CAD build for the part. Positions are in the model's coordinates, mm. Face numbers are marked on the shaded views. A direction names the side the tool comes from. Coordinates: 2 decimals unless noted, no trailing zeros. Loops run counter-clockwise (first coordinate to the right, second up) from the corner with the lowest first, then second, coordinate; pieces in that order, holes last. Notation, with made-up numbers: (-17.75, 53.5) -> (41.25, 53.5) arc R21 cw to (41.25, 92.5) -> close; hole circle Ø1 at (68.5, 66). An arc over 180 degrees is marked (long way). Write each question's results on one line, items separated by ' | '.
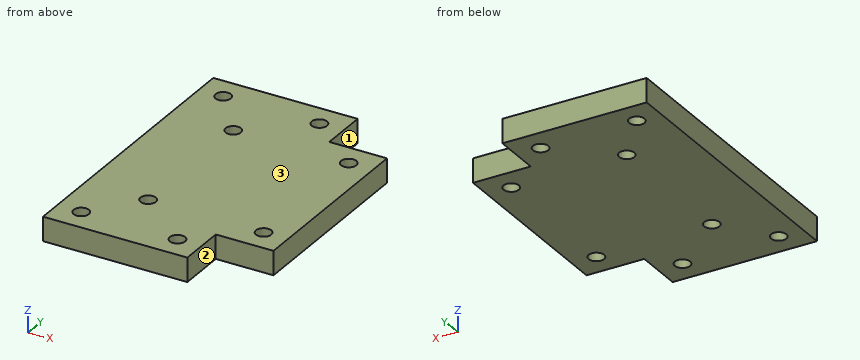
from build123d import *

# Parameters (mm, degrees)
EXTRUDE_1_DEPTH     = 5
SKETCH_5_R          = 1.6
CUT_EXTRUDE_1_DEPTH = 329.148213465
SKETCH_6_W          = 3
SKETCH_6_H          = 30
CUT_EXTRUDE_2_DEPTH = 329.148213465
SKETCH_7_W          = 3
SKETCH_7_H          = 10
CUT_EXTRUDE_3_DEPTH = 329.148213465
SKETCH_8_W          = 15
SKETCH_8_H          = 3
CUT_EXTRUDE_4_DEPTH = 329.148213465
SKETCH_9_W          = 30
SKETCH_9_H          = 0.36
EXTRUDE_2_DEPTH     = 5
SKETCH_11_W         = 200
SKETCH_11_H         = 355
SKETCH_11_W_2       = 46
SKETCH_11_H_2       = 60
CUT_EXTRUDE_5_DEPTH = 329.148213465
CUT_EXTRUDE_7_DEPTH = 221.184013952
SKETCH_13_R         = 1.6
CUT_EXTRUDE_8_DEPTH = 220.018264079


with BuildPart() as part:
    # 草图3 → 凸台-拉伸1 (new body)
    with BuildSketch(Plane.XY):
        Polygon((-10, 267.5), (190, 267.5), (190, 230), (160, 230), (160, 130), (190, 130), (190, 50), (160, 50), (160, -50), (190, -50), (190, -87.5), (-10, -87.5), (-10, -50), (20, -50), (20, 50), (-10, 50), (-10, 130), (20, 130), (20, 230), (-10, 230), align=None)
    extrude(amount=EXTRUDE_1_DEPTH)

    # 草图5 → 切除-拉伸1 (cut, through all)
    with BuildSketch(Plane.XY.offset(5)):
        with Locations((33, 195)):
            Circle(SKETCH_5_R)
        with Locations((57, 195)):
            Circle(SKETCH_5_R)
        with Locations((33, 165)):
            Circle(SKETCH_5_R)
        with Locations((57, 165)):
            Circle(SKETCH_5_R)
        with Locations((123, 195)):
            Circle(SKETCH_5_R)
        with Locations((147, 195)):
            Circle(SKETCH_5_R)
        with Locations((123, 165)):
            Circle(SKETCH_5_R)
        with Locations((147, 165)):
            Circle(SKETCH_5_R)
        with Locations((33, 15)):
            Circle(SKETCH_5_R)
        with Locations((57, 15)):
            Circle(SKETCH_5_R)
        with Locations((33, -15)):
            Circle(SKETCH_5_R)
        with Locations((57, -15)):
            Circle(SKETCH_5_R)
        with Locations((123, 15)):
            Circle(SKETCH_5_R)
        with Locations((147, 15)):
            Circle(SKETCH_5_R)
        with Locations((123, -15)):
            Circle(SKETCH_5_R)
        with Locations((147, -15)):
            Circle(SKETCH_5_R)
    extrude(amount=-CUT_EXTRUDE_1_DEPTH, mode=Mode.SUBTRACT)

    # 草图6 → 切除-拉伸2 (cut, through all)
    with BuildSketch(Plane.XY.offset(5)):
        with Locations((-8.5, 90)):
            Rectangle(SKETCH_6_W, SKETCH_6_H)
        with Locations((188.5, 90)):
            Rectangle(SKETCH_6_W, SKETCH_6_H)
    extrude(amount=-CUT_EXTRUDE_2_DEPTH, mode=Mode.SUBTRACT)

    # 草图7 → 切除-拉伸3 (cut, through all)
    with BuildSketch(Plane.XY.offset(5)):
        with Locations((-8.5, 248.75)):
            Rectangle(SKETCH_7_W, SKETCH_7_H)
        with Locations((188.5, 248.75)):
            Rectangle(SKETCH_7_W, SKETCH_7_H)
        with Locations((-8.5, -68.75)):
            Rectangle(SKETCH_7_W, SKETCH_7_H)
        with Locations((188.5, -68.75)):
            Rectangle(SKETCH_7_W, SKETCH_7_H)
    extrude(amount=-CUT_EXTRUDE_3_DEPTH, mode=Mode.SUBTRACT)

    # 草图8 → 切除-拉伸4 (cut, through all)
    with BuildSketch(Plane.XY.offset(5)):
        with Locations((17.5, -86)):
            Rectangle(SKETCH_8_W, SKETCH_8_H)
        with Locations((52.5, -86)):
            Rectangle(SKETCH_8_W, SKETCH_8_H)
        with Locations((127.5, -86)):
            Rectangle(SKETCH_8_W, SKETCH_8_H)
        with Locations((162.5, -86)):
            Rectangle(SKETCH_8_W, SKETCH_8_H)
    extrude(amount=-CUT_EXTRUDE_4_DEPTH, mode=Mode.SUBTRACT)

    # 草图9 → 凸台-拉伸2 (add)
    with BuildSketch(Plane.XY.offset(5)):
        with Locations((5, 229.82)):
            Rectangle(SKETCH_9_W, SKETCH_9_H)
        with Locations((175, 229.82)):
            Rectangle(SKETCH_9_W, SKETCH_9_H)
    extrude(amount=-EXTRUDE_2_DEPTH)

    # 草图11 → 切除-拉伸5 (cut, through all)
    with BuildSketch(Plane.XY.offset(5)):
        with Locations((90, 90)):
            Rectangle(SKETCH_11_W, SKETCH_11_H)
        with Locations((43, 180)):
            Rectangle(SKETCH_11_W_2, SKETCH_11_H_2, mode=Mode.SUBTRACT)
    extrude(amount=-CUT_EXTRUDE_5_DEPTH, mode=Mode.SUBTRACT)

    # 草图14 → 切除-拉伸7 (cut, through all)
    with BuildSketch(Plane(origin=(0, 0, 0), x_dir=(-1, 0, 0), z_dir=(0, 0, -1))):
        Polygon((-66, 150), (-50, 150), (-50, 160), (-62, 160), (-62, 200), (-50, 200), (-50, 210), (-66, 210), (-66, 200), (-66, 160), align=None)
    extrude(amount=-CUT_EXTRUDE_7_DEPTH, mode=Mode.SUBTRACT)

    # 草图13 → 切除-拉伸8 (cut, through all)
    with BuildSketch(Plane.XY.offset(5)):
        with Locations((45, 205)):
            Circle(SKETCH_13_R)
        with Locations((25, 155)):
            Circle(SKETCH_13_R)
        with Locations((25, 205)):
            Circle(SKETCH_13_R)
        with Locations((45, 155)):
            Circle(SKETCH_13_R)
    extrude(amount=-CUT_EXTRUDE_8_DEPTH, mode=Mode.SUBTRACT)


solid = part.part
1) Slice it at C-C (z = 2.5). Count the separate pieces of the cut face and the enclosed holes in it, then the cut area to 3 significant figures.
Outcome:
separate pieces: 1 | enclosed holes: 8 | area: 2,220 mm^2
2) Drill centre lines: L1, parallel to X at y = 195, z = 1.8; L2, parallel to Y at x = 57, z = 0.65; L3, parallel to Y at x = 25, z = 3.7. Where is each one in solid material? Low to high. Write a range as from..to.
Outcome:
L1: x = 20..31.4, 34.6..55.4, 58.6..62 | L2: y = 160..163.4, 166.6..193.4, 196.6..200 | L3: y = 150..153.4, 156.6..203.4, 206.6..210
3) Slice it at B-B (y = 155). Write the cut outline in (x, z).
Outcome:
outline: (20, 0) -> (23.4, 0) -> (23.4, 5) -> (20, 5) -> close; (26.6, 0) -> (43.4, 0) -> (43.4, 5) -> (26.6, 5) -> close; (46.6, 0) -> (50, 0) -> (50, 5) -> (46.6, 5) -> close
4) Pin check, flat tips, straight feed: pin 1 (2.5 mm diameter, centred on x = 58.5, z = 3.5, fed in from +Y); pin 2 (12 mm diameter, centred on x = 33.5, y = 174, fed in from -Z); pin 3 (2.5 mm diameter, centred on x = 58, z = 2.5, fed in from -Y). Stop position of each tip, or through.
Outcome:
pin 1: stops at y = 200 | pin 2: stops at z = 0 | pin 3: stops at y = 160
5) Which spindle directions (+Z, -Z, +X, -X, +Y, -Y) get a long thin tool onto all of the face, cutting with end or side? Do the marked faces 1, 2 and 3. Say none if no direction does.
Outcome:
face 1: +Z, -Z, +X, +Y | face 2: +Z, -Z, +X, -Y | face 3: +Z, +X, -X, +Y, -Y
6) Slice it at A-A (x = 25). Write the cut outline in (y, z), then the cut area to 3 significant figures.
Outcome:
outline: (150, 0) -> (153.4, 0) -> (153.4, 5) -> (150, 5) -> close; (156.6, 0) -> (203.4, 0) -> (203.4, 5) -> (156.6, 5) -> close; (206.6, 0) -> (210, 0) -> (210, 5) -> (206.6, 5) -> close | area: 268 mm^2
